```python
from build123d import *

# Parameters (mm, degrees)
PAD_DEPTH       = 3
SKETCH001_W     = 3
SKETCH001_H     = 26
PAD001_DEPTH    = 24
SKETCH002_R     = 2
POCKET_DEPTH    = 3
PAD002_DEPTH    = 3
SKETCH004_R     = 1.5
POCKET001_DEPTH = 30.001


with BuildPart() as part:
    # Sketch → Pad (new body)
    with BuildSketch(Plane.XY):
        with BuildLine():
            ThreePointArc((33.5, 33.5), (0, 0), (33.5, -33.5))
            Line((33.5, -33.5), (33.5, -59.5))
            Line((33.5, -59.5), (8, -59.5))
            Line((8, -59.5), (8, -35.24202))
            ThreePointArc((33.5, 43.5), (-7.884042, 13.401905), (8, -35.24202))
            Line((33.5, 33.5), (33.5, 43.5))
        make_face()
    extrude(amount=PAD_DEPTH)

    # Sketch001 → Pad001 (new body)
    with BuildSketch(Plane.XY.offset(3)):
        with Locations((32, -46.5)):
            Rectangle(SKETCH001_W, SKETCH001_H)
    extrude(amount=PAD001_DEPTH)

    # Sketch002 → Pocket (cut)
    with BuildSketch(Plane.YZ.offset(33.5)):
        with Locations((-36.5, 21)):
            Circle(SKETCH002_R)
        with Locations((-36.5, 15)):
            Circle(SKETCH002_R)
        with Locations((-36.5, 9)):
            Circle(SKETCH002_R)
    extrude(amount=-POCKET_DEPTH, mode=Mode.SUBTRACT)

    # Sketch003 → Pad002 (new body)
    with BuildSketch(Plane.XY.offset(27)):
        with BuildLine():
            Line((33.5, 43.5), (33.5, 33.5))
            ThreePointArc((33.5, 33.5), (0, 0), (33.5, -33.5))
            Line((33.5, -33.5), (33.5, -59.5))
            Line((8, -59.5), (33.5, -59.5))
            Line((8, -35.24202), (8, -59.5))
            ThreePointArc((33.5, 43.5), (-7.884042, 13.401905), (8, -35.24202))
        make_face()
    extrude(amount=PAD002_DEPTH)

    # Sketch004 → Pocket001 (cut, through all)
    with BuildSketch(Plane(origin=(0, 0, 0), x_dir=(1, 0, 0), z_dir=(0, 0, -1))):
        with Locations((1.962646, 22.082693)):
            Circle(SKETCH004_R)
        with Locations((8.68646, -29.464001)):
            Circle(SKETCH004_R)
        with Locations((0.158022, -19.25)):
            Circle(SKETCH004_R)
    extrude(amount=-POCKET001_DEPTH, mode=Mode.SUBTRACT)


solid = part.part
```
The listing builds one solid part. Answer for the finished solid, in the listing's coordinates (mm). A direction names the side the tool comes from. Coordinates: 2 decimals unless noted, no trailing zeros. Write each loop counter-clockwise with the first axis right and the second up, starting at its lowest first coordinate (ties: lowest second). Pieces come first, ordered by that corner, then holes. Notation, with made-up numbers: (-36, 35) - (-12, 35) arc R25 ccw to (-12, 66) - close; hole circle Ø5 at (-28, 12.5). An arc over 180 degrees is marked (long way). Return JSON: item names as keys, results as strings. Group by question number.
Q1. The part is cut by section B-B on y = 0. Write down the section's boundary in (x, z).
Q2. The part is cut by section C-C on x = 12.5. Write down the section's boundary in (y, z), and give its area (3 significant figures).
Q3. Which of the six approach directions +Z, -Z, +X, -X, +Y, -Y give full straight-line access (tool end or side, diameter ignored) to faces 4 (the flat face through (8, -48, 1)), 5 (the flat face through (31, -59.5, 16))?
Q4. Find the intervals of material crossed by line 1 along Z through (x, y) = (31.35, -36.5); line 2 along Z through (x, y) = (15, -41.5); line 3 along X through (y, z) = (-35, 12.5), in increasing order. Write a range as [from, to].
Q5. Flat-ended cylindrical pins translate along their axes: pin 1 Ø2.5 at (y, z) = (-51.5, 28.5) entering from -X; pin 2 Ø12 at (x, z) = (-3.5, 4.5) entering from +Y. Find the tip coordinate at first contact, or state that the pin passes through.
Q6. The part is cut by section D-D on y = -36.5. Write down the section's boundary in (x, z), and give its area (3 significant figures).
Q7. The part is cut by section A-A on z = 15. Write down the section's boundary in (x, y), and give its area (3 significant figures).
Q8. For a pull along X with two mould halves and no side action, classify faces 1 (the cylindrical face through (-7.64, 14.13, 28.48)), 2 (the cylindrical face through (-0.037, 17.763, 28.479)), 3 (the flat face through (2, -15, 27)) as +X half, -X half, draft (parallel to the pull), parting line (faces both ways), or undercut.
Evaluation:
{
 "1": {"outline": "(-10, 0) - (0, 0) - (0, 3) - (-10, 3) - close; (-10, 27) - (0, 27) - (0, 30) - (-10, 30) - close"},
 "2": {"outline": "(-59.5, 0) - (-26.1, 0) - (-26.1, 3) - (-59.5, 3) - close; (-59.5, 27) - (-26.1, 27) - (-26.1, 30) - (-59.5, 30) - close; (26.1, 0) - (38.1, 0) - (38.1, 3) - (26.1, 3) - close; (26.1, 27) - (38.1, 27) - (38.1, 30) - (26.1, 30) - close", "area": "272 mm2"},
 "3": {"face 4": "+Z, -Z, -X, -Y", "face 5": "+Z, -Z, +X, -X, -Y"},
 "4": {"line 1": "z = [0, 7], [11, 13], [17, 19], [23, 30]", "line 2": "z = [0, 3], [27, 30]", "line 3": "x = [30.5, 33.5]"},
 "5": {"pin 1": "stops at x = 8", "pin 2": "stops at y = 30.32"},
 "6": {"outline": "(8, 0) - (33.5, 0) - (33.5, 7) - (30.5, 7) - (30.5, 3) - (8, 3) - close; (8, 27) - (30.5, 27) - (30.5, 23) - (33.5, 23) - (33.5, 30) - (8, 30) - close; (30.5, 11) - (33.5, 11) - (33.5, 13) - (30.5, 13) - close; (30.5, 17) - (33.5, 17) - (33.5, 19) - (30.5, 19) - close", "area": "189 mm2"},
 "7": {"outline": "(30.5, -59.5) - (33.5, -59.5) - (33.5, -38.5) - (30.5, -38.5) - close; (30.5, -34.5) - (33.5, -34.5) - (33.5, -33.5) - (30.5, -33.5) - close", "area": "66.0 mm2"},
 "8": {"face 1": "-X half", "face 2": "undercut", "face 3": "draft"}
}
